Check sheet for the modelled part. Datum: model origin and axes. Units: mm. A direction names the side the tool comes from. Give positions to 0.01 mm unless a question says otherwise; leave off trailing zeros. Write each loop counter-clockwise with the first axis right and the second up, starting at its lowest first coordinate (ties: lowest second). Pieces come first, ordered by that corner, then holes.
from build123d import *

# Parameters (mm, degrees)
SKETCH1_W           = 48
SKETCH1_H           = 35
BOSS_EXTRUDE1_DEPTH = 65
SKETCH2_R           = 7.5
SKETCH2_R_2         = 3.5
CUT_EXTRUDE1_DEPTH  = 89.056799851
SKETCH3_W           = 14
SKETCH3_H           = 65
CUT_EXTRUDE2_DEPTH  = 12.5
SKETCH4_W           = 14
SKETCH4_H           = 55
CUT_EXTRUDE3_DEPTH  = 12
CUT_EXTRUDE4_DEPTH  = 60
SKETCH6_R           = 7.25
CUT_EXTRUDE5_DEPTH  = 5
SKETCH7_W           = 11
SKETCH7_H           = 35
CUT_EXTRUDE6_DEPTH  = 89.056799851
SKETCH8_R           = 4
CUT_EXTRUDE7_DEPTH  = 30
SKETCH9_W           = 38
SKETCH9_H           = 35
CUT_EXTRUDE8_DEPTH  = 10
FILLET1_R           = 3
SKETCH11_W          = 21
SKETCH11_H          = 65
BOSS_EXTRUDE2_DEPTH = 25
FILLET2_R           = 10
CUT_EXTRUDE9_DEPTH  = 104.821962994
FILLET3_R           = 2
SKETCH13_W          = 11
SKETCH13_H          = 35
CUT_EXTRUDE10_DEPTH = 104.821962994
CUT_EXTRUDE11_DEPTH = 104.821962994
SKETCH16_R          = 1.5
CUT_EXTRUDE13_DEPTH = 104.821962994
CUT_EXTRUDE14_DEPTH = 3
FILLET4_R           = 2


with BuildPart() as part:
    # Sketch1 → Boss-Extrude1 (new body)
    with BuildSketch(Plane(origin=(0, 0, 0), x_dir=(1, 0, 0), z_dir=(0, 1, 0))):
        with Locations((24, 17.5)):
            Rectangle(SKETCH1_W, SKETCH1_H)
    extrude(amount=BOSS_EXTRUDE1_DEPTH)

    # Sketch2 → Cut-Extrude1 (cut, through all)
    with BuildSketch(Plane(origin=(0, 65, 0), x_dir=(1, 0, 0), z_dir=(0, 1, 0))):
        with Locations(Location((36, 11, 0), (0, 0, 270))):
            Circle(SKETCH2_R)
        with Locations(Location((20.5, 11, 0), (0, 0, 270))):
            Circle(SKETCH2_R_2)
    extrude(amount=-CUT_EXTRUDE1_DEPTH, mode=Mode.SUBTRACT)

    # Sketch3 → Cut-Extrude2 (cut)
    with BuildSketch(Plane.ZY):
        with Locations((-7, 32.5)):
            Rectangle(SKETCH3_W, SKETCH3_H)
    extrude(amount=-CUT_EXTRUDE2_DEPTH, mode=Mode.SUBTRACT)

    # Sketch4 → Cut-Extrude3 (cut)
    with BuildSketch(Plane.ZY.offset(-12.5)):
        with Locations((-7, 27.5)):
            Rectangle(SKETCH4_W, SKETCH4_H)
    extrude(amount=-CUT_EXTRUDE3_DEPTH, mode=Mode.SUBTRACT)

    # Sketch5 → Cut-Extrude4 (cut)
    with BuildSketch(Plane.XZ):
        Polygon((25.215019923, -14.528255535), (25.913068886, -8.680800735), (21.198048963, -5.152545199), (15.784980077, -7.471744465), (15.086931114, -13.319199265), (19.801951037, -16.847454801), align=None)
    extrude(amount=-CUT_EXTRUDE4_DEPTH, mode=Mode.SUBTRACT)

    # Sketch6 → Cut-Extrude5 (cut)
    with BuildSketch(Plane(origin=(0, 0, 0), x_dir=(-1, 0, 0), z_dir=(0, -1, 0))):
        with Locations((-20.5, 11)):
            Circle(SKETCH6_R)
    extrude(amount=-CUT_EXTRUDE5_DEPTH, mode=Mode.SUBTRACT)

    # Sketch7 → Cut-Extrude6 (cut, through all)
    with BuildSketch(Plane.ZY):
        with Locations((-24.5, 32.5)):
            Rectangle(SKETCH7_W, SKETCH7_H)
    extrude(amount=-CUT_EXTRUDE6_DEPTH, mode=Mode.SUBTRACT)

    # Sketch8 → Cut-Extrude7 (cut)
    with BuildSketch(Plane.ZY):
        with Locations((-24.5, 58)):
            Circle(SKETCH8_R)
        with Locations((-24.5, 7)):
            Circle(SKETCH8_R)
    extrude(amount=-CUT_EXTRUDE7_DEPTH, mode=Mode.SUBTRACT)

    # Sketch9 → Cut-Extrude8 (cut)
    with BuildSketch(Plane(origin=(0, 0, -35), x_dir=(-1, 0, 0), z_dir=(0, 0, -1))):
        with Locations((-24, 32.5)):
            Rectangle(SKETCH9_W, SKETCH9_H)
    extrude(amount=-CUT_EXTRUDE8_DEPTH, mode=Mode.SUBTRACT)

    # Fillet1
    fillet1_edges = [part.edges().sort_by_distance(p)[0] for p in [
        (0, 32.5, -14),
        (12.5, 60, 0),
        (24.5, 27.5, 0),
        (0, 32.5, -35),
    ]]
    fillet(fillet1_edges, radius=FILLET1_R)

    # Sketch11 → Boss-Extrude2 (add)
    with BuildSketch(Plane(origin=(48, 0, 0), x_dir=(0, 0, -1), z_dir=(1, 0, 0))):
        with Locations((24.5, 32.5)):
            Rectangle(SKETCH11_W, SKETCH11_H)
    extrude(amount=BOSS_EXTRUDE2_DEPTH)

    # Fillet2
    fillet2_edges = [part.edges().sort_by_distance(p)[0] for p in [
        (48, 32.5, 0),
    ]]
    fillet(fillet2_edges, radius=FILLET2_R)

    # Sketch12 → Cut-Extrude9 (cut, through all)
    with BuildSketch(Plane(origin=(0, 65, 0), x_dir=(1, 0, 0), z_dir=(0, 1, 0))):
        Polygon((36, 0), (36, 3.5), (38, 3.771583853), (38, 0), align=None)
    extrude(amount=-CUT_EXTRUDE9_DEPTH, mode=Mode.SUBTRACT)

    # Fillet3
    # the kernel refuses this fillet: 2 mm, written as the material it takes off along each edge
    with BuildSketch(Plane(origin=(38, -6.300214624, 0), x_dir=(0.9920296962671666, 0, -0.12600429248272813), z_dir=(0, 1, 0))) as fillet3_piece_1:
        with BuildLine():
            CenterArc((2.268077265, 1.984059393), FILLET3_R, 172.761243907, 104.477512186)
            Line((0.284017872, 2.236067977), (0, 0))
            ThreePointArc((0, 0), (1.260042925, -0.079703037), (2.52008585, 0))
        make_face()
    extrude(amount=77.600429248, mode=Mode.SUBTRACT)
    with BuildSketch(Plane(origin=(36, 70, 0), x_dir=(-1, 0, 0), z_dir=(0, -1, 0))) as fillet3_piece_2:
        with BuildLine():
            CenterArc((FILLET3_R, FILLET3_R), FILLET3_R, 180, 90)
            Line((0, FILLET3_R), (0, 0))
            Line((0, 0), (FILLET3_R, 0))
        make_face()
    extrude(amount=75, mode=Mode.SUBTRACT)
    with BuildSketch(Plane(origin=(36, 69.467719526, -3.5), x_dir=(0, 0, 1), z_dir=(0, -1, 0))) as fillet3_piece_3:
        with BuildLine():
            CenterArc((1.787087811, 2), FILLET3_R, 192.153197469, 77.846802531)
            ThreePointArc((-0.168088571, 1.578947368), (-0.042140531, 0.793934594), (0, 0))
            Line((0, 0), (1.787087811, 0))
        make_face()
    extrude(amount=73.935439053, mode=Mode.SUBTRACT)
    with BuildSketch(Plane(origin=(38, 68.471069556, -3.771583853), x_dir=(0, 0, 1), z_dir=(0, -1, 0))) as fillet3_piece_4:
        with BuildLine():
            CenterArc((1.388427822, -2), FILLET3_R, 90, 65.09893763)
            ThreePointArc((-0.425644592, -1.157894737), (-0.188974611, -0.587713829), (0, 0))
            Line((0, 0), (1.388427822, 0))
        make_face()
    extrude(amount=71.942139112, mode=Mode.SUBTRACT)

    # Sketch13 → Cut-Extrude10 (cut, through all)
    with BuildSketch(Plane(origin=(73, 0, 0), x_dir=(0, 0, -1), z_dir=(1, 0, 0))):
        with Locations((24.5, 32.5)):
            Rectangle(SKETCH13_W, SKETCH13_H)
    extrude(amount=-CUT_EXTRUDE10_DEPTH, mode=Mode.SUBTRACT)

    # Sketch14 → Cut-Extrude11 (cut, through all)
    with BuildSketch(Plane(origin=(0, 0, -35), x_dir=(-1, 0, 0), z_dir=(0, 0, -1))):
        Polygon((-73, 65), (-58, 65), (-73, 55), align=None)
        Polygon((-73, 0), (-58, 0), (-73, 10), align=None)
    extrude(amount=-CUT_EXTRUDE11_DEPTH, mode=Mode.SUBTRACT)

    # Sketch16 → Cut-Extrude13 (cut, through all)
    with BuildSketch(Plane(origin=(0, 0, -35), x_dir=(-1, 0, 0), z_dir=(0, 0, -1))):
        with Locations((-63, 32.5)):
            Circle(SKETCH16_R)
    extrude(amount=-CUT_EXTRUDE13_DEPTH, mode=Mode.SUBTRACT)

    # Sketch17 → Cut-Extrude14 (cut)
    with BuildSketch(Plane.XY.offset(-14)):
        Polygon((60.700217219, 35.090559623), (59.606618166, 31.8036095), (61.906400947, 29.213049877), (65.299782781, 29.909440377), (66.393381834, 33.1963905), (64.093599053, 35.786950123), align=None)
    extrude(amount=-CUT_EXTRUDE14_DEPTH, mode=Mode.SUBTRACT)

    # Fillet4
    fillet4_edges = [part.edges().sort_by_distance(p)[0] for p in [
        (65.5, 5, -35),
        (65.5, 5, -14),
        (65.5, 60, -35),
        (65.5, 60, -14),
        (73, 32.5, -14),
        (73, 32.5, -35),
        (58, 0, -24.5),
        (73, 10, -24.5),
        (73, 55, -24.5),
        (58, 65, -24.5),
    ]]
    fillet(fillet4_edges, radius=FILLET4_R)


solid = part.part
1) Gauge pin test, flat ends, axial feed: pin 1 (6 mm diameter, centred on x = 12.5, y = 46, fed in from +Z); pin 2 (6.5 mm diameter, centred on y = 58, z = -24.5, fed in from -X); pin 3 (1.8 mm diameter, centred on x = 63, y = 32.5, fed in from +Z); pin 4 (4 mm diameter, centred on x = 23, z = -10.5, fed in from -Y). Record the tip position at first contact, or that the pin passes through.
2) Draft check along X on faces 5 (the cylindrical face through (25.4, 27.88, -0.86)), 6 (the flat face through (43, 32, -33)), 7 (the flat face through (28, 0, -21)), 8 (the cylindrical face through (25.062, 2.465, -16.635)). Enter one of: +X half, -X half, draft (parallel to the pull), parting line (faces both ways), or undercut.
3) Sectioned sample at C-C on y = 12. Record the boundary of the cut face in (x, z).
4) Scan lines: L1, parallel to X at y = 42, z = -15; L2, parallel to X at y = 3.1, z = -11; L3, parallel to Z at x = 53, y = 39.5. Record each from-to range of solid material in increasing order.
5) Sectioned sample at A-A on y = 47. Give the number of separate pieces and of enclosed holes in the cut face, then the cut area to 3 significant figures.
6) Sectioned sample at B-B on z = -11. Record the boundary of the cut face in (x, y), then the cut area to 3 significant figures.
7) Access from +Z, -Z, +X, -X, +Y, -Y to the whole of each face (thin tool, end or side, straight path). Record for faces 1 (the flat face through (59, 32, -14)), 2 (the flat face through (5, 32, -33)), 3 (the flat face through (36, 32, -19)), 4 (the flat face through (63.579, 29.556, -15.479)).
Answers below:
1. pin 1: stops at z = -14
1. pin 2: stops at x = 30
1. pin 3: passes through
1. pin 4: stops at y = 60
2. face 5: -X half
2. face 6: undercut
2. face 7: draft
2. face 8: undercut
3. outline: (0, -32) arc R3 ccw to (3, -35) - (71, -35) arc R2 ccw to (73, -33) - (73, -16) arc R2 ccw to (71, -14) - (48, -14) - (48, -10) arc R10 ccw to (40.5, -0.32) arc R2 ccw to (38, -2.25) - (38, -2.38) arc R2 ccw to (39.16, -4.2) arc R7.5 cw (long way) to (34.42, -3.67) arc R2 ccw to (35.99, -1.86) arc R2 ccw to (34, 0) - (27.5, 0) arc R3 ccw to (24.5, -3) - (24.5, -7.62) - (25.91, -8.68) - (25.22, -14.53) - (19.8, -16.85) - (16, -14) - (3, -14) arc R3 ccw to (0, -17) - close
4. L1: x = 0.76 to 17.33, 24.11 to 29.66, 42.34 to 72.73
4. L2: x = 27.75 to 28.5, 43.5 to 48
4. L3: z = -35 to -30, -19 to -14
5. separate pieces: 3
5. enclosed holes: 0
5. area: 632 mm2
6. outline: (12.5, 55) - (15.36, 55) - (15.36, 60) - (17, 60) - (17, 65) - (12.5, 65) - close; (24, 60) - (25.64, 60) - (25.64, 5) - (27.75, 5) - (27.75, 0) - (28.5, 0) - (28.5, 65) - (24, 65) - close; (43.5, 0) - (48, 0) - (48, 65) - (43.5, 65) - close
6. area: 513 mm2
7. face 1: +Z, +X, +Y, -Y
7. face 2: -Z
7. face 3: +X, -X
7. face 4: +Z
